Work out the finished part from the listing and answer in its coordinate system (mm). Coordinates: 2 decimals unless noted, no trailing zeros. Write each loop counter-clockwise with the first axis right and the second up, starting at its lowest first coordinate (ties: lowest second). Pieces come first, ordered by that corner, then holes. Notation, with made-up numbers: (42.5, -33) - (71.5, -33) arc R20 cw to (71.5, 3) - close; hole circle Ø9 at (40, 5.5). An arc over 180 degrees is marked (long way). Use one line per item in the form item = value. Start each with the question number.
Item 1: Consider probe 1 along Y at (x, z) = (62.5, 3.85) (3 decimals); probe 2 along Y at (x, z) = (42.5, 4.75) (3 decimals); probe 3 along X at (y, z) = (2.5, 3.8). Determine where each line is inside the solid, lowest interval first.
Item 2: A cutting plane is placed at A-A (y = -59.5). Write down the section's boundary in (x, z), then the cut area to 3 significant figures.
Item 3: A cutting plane is placed at B-B (x = 72.5). Write down the section's boundary in (y, z), then the cut area to 3 significant figures.
Item 4: Given pin 1 (3 mm diameter, centred on x = 72.5, y = -59.5, fed in from +Z), flat-ended and moving along its own axis, determine where the tip first touches the part or whether it passes through.
from build123d import *

# Parameters (mm, degrees)
ESQUISSE1_W             = 155
ESQUISSE1_H             = 140
ESQUISSE1_R             = 5
ESQUISSE1_R_2           = 2.5
BOSS_EXTRU_1_DEPTH      = 6
ESQUISSE6_R             = 1.5
ENL_V_MAT_EXTRU_1_DEPTH = 6


with BuildPart() as part:
    # Esquisse1 → Boss.-Extru.1 (new body)
    with BuildSketch(Plane.XY):
        with Locations((0, 5.5)):
            Rectangle(ESQUISSE1_W, ESQUISSE1_H)
        with Locations((42.5, -44.9)):
            Circle(ESQUISSE1_R, mode=Mode.SUBTRACT)
        with Locations((42.5, 55.875)):
            Circle(ESQUISSE1_R, mode=Mode.SUBTRACT)
        with Locations((-72.5, -59.5)):
            Circle(ESQUISSE1_R_2, mode=Mode.SUBTRACT)
        with Locations((-72.5, 70.5)):
            Circle(ESQUISSE1_R_2, mode=Mode.SUBTRACT)
        with Locations((72.5, -59.5)):
            Circle(ESQUISSE1_R_2, mode=Mode.SUBTRACT)
        with Locations((72.5, 70.5)):
            Circle(ESQUISSE1_R_2, mode=Mode.SUBTRACT)
    extrude(amount=BOSS_EXTRU_1_DEPTH)

    # Esquisse6 → Enlèv. mat.-Extru.1 (cut)
    with BuildSketch(Plane.XY.offset(6)):
        with Locations((-17.5, 12.875)):
            Circle(ESQUISSE6_R)
        with Locations((22.5, 12.875)):
            Circle(ESQUISSE6_R)
        with Locations((62.5, 12.875)):
            Circle(ESQUISSE6_R)
        with Locations((62.5, 1.875)):
            Circle(ESQUISSE6_R)
        with Locations((22.5, 1.875)):
            Circle(ESQUISSE6_R)
        with Locations((-17.5, 1.875)):
            Circle(ESQUISSE6_R)
    extrude(amount=-ENL_V_MAT_EXTRU_1_DEPTH, mode=Mode.SUBTRACT)


solid = part.part
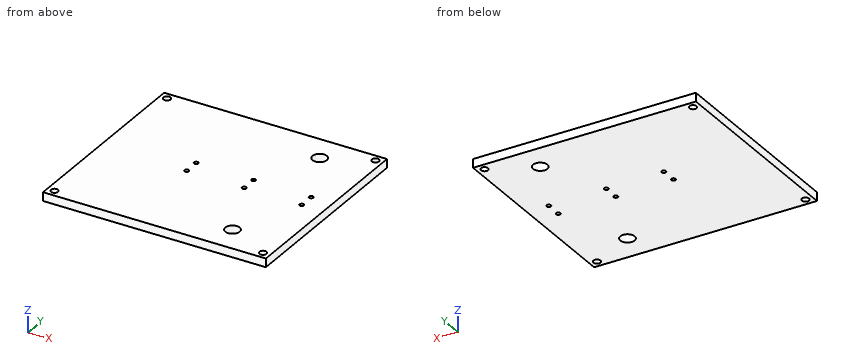
Answer:
q1.probe_1 = -64.5 to 0.375, 3.375 to 11.375, 14.375 to 75.5
q1.probe_2 = -64.5 to -49.9, -39.9 to 50.875, 60.875 to 75.5
q1.probe_3 = -77.5 to -18.86, -16.14 to 21.14, 23.86 to 61.14, 63.86 to 77.5
q2.outline = (-77.5, 0) - (-75, 0) - (-75, 6) - (-77.5, 6) - close; (-70, 0) - (70, 0) - (70, 6) - (-70, 6) - close; (75, 0) - (77.5, 0) - (77.5, 6) - (75, 6) - close
q2.area = 870 mm²
q3.outline = (-64.5, 0) - (-62, 0) - (-62, 6) - (-64.5, 6) - close; (-57, 0) - (68, 0) - (68, 6) - (-57, 6) - close; (73, 0) - (75.5, 0) - (75.5, 6) - (73, 6) - close
q3.area = 780 mm²
q4.pin_1 = through
